from build123d import *

# Parameters (mm, degrees)
SKETCH1_R           = 14.2875
BOSS_EXTRUDE1_DEPTH = 3.9751
SKETCH2_R           = 12.7
SKETCH2_R_2         = 8.73125
CUT_EXTRUDE1_DEPTH  = 0.508


with BuildPart() as part:
    # Sketch1 → Boss-Extrude1 (new body, symmetric)
    with BuildSketch(Plane.XY):
        Circle(SKETCH1_R)
        Polygon((7.332348419, 0), (3.666174209, 6.35), (-3.666174209, 6.35), (-7.332348419, 0), (-3.666174209, -6.35), (3.666174209, -6.35), align=None, mode=Mode.SUBTRACT)
    extrude(amount=BOSS_EXTRUDE1_DEPTH, both=True)

    # Sketch2 → Cut-Extrude1 (cut)
    with BuildSketch(Plane.XY.offset(3.9751)):
        Circle(SKETCH2_R)
        Circle(SKETCH2_R_2, mode=Mode.SUBTRACT)
    cut_extrude1 = extrude(amount=-CUT_EXTRUDE1_DEPTH, mode=Mode.SUBTRACT)

    # Mirror1: Cut-Extrude1 across plane
    add(cut_extrude1.mirror(Plane.XY), mode=Mode.SUBTRACT)


solid = part.part
For this review, take the finished solid that the model builds, in its own axes (mm). A direction names the side the tool comes from. Round coordinates to 2 decimals unless told otherwise and drop trailing zeros. Order: outer loops, then holes, each group sorted by start corner. A loop starts at its lowest first (then second) coordinate and runs counter-clockwise, first axis right, second up. Notation, with made-up numbers: M 71.25,40 L 102.25,40 A17 cw 102.25,51 Z; hole C 25.5,65 d8. An arc over 180 degrees is marked long. Write each question's results on one line, items separated by ' | '. Start each with the question number.
1. To check wall thickness, follow L1, parallel to Y at x = 0, z = 3.85; L2, parallel to Y at x = 0, z = -0.25; L3, parallel to X at y = 2.25, z = -3.5. State the ranges of each line that lie inside material, in increasing order. Write a range as [from, to].
2. Clearance check with flat-ended pins moving along their axes: pin 1 Ø4 at (y, z) = (-3.5, -2.5) entering from -X; pin 2 Ø3 at (x, z) = (-9, -1) entering from -Y. State where each tip first meets the part, or that it passes through.
3. Draft analysis for pull direction Y (two halves, no side actions). For faces 4 (the face through (0, -6.35, 0)), 5 (the face through (5.1, -4.5, -3.975)), 6 (the face through (-14.274, 0.628, 0.056)), state which applies: pulls with the +Y half, pulls with the -Y half, needs draft (parallel to the pull), parting line crosses it, or undercut.
4. Add section A-A (x = 0). State the section outline as (y, z) points.
5. Add section C-C (y = 0.75). State the section outline as (x, z) points, then the cut area to 3 significant figures.
6. Tool access review of faces 1 (the face through (3, 9, 3.467)), 2 (the face through (3, 9, -3.467)), 3 (the face through (-5.474, 3.219, 0.056)): name each direction out of +Z, -Z, +X, -X, +Y, -Y from which nothing blocks a thin tool from reaching the whole face with its end or side.
7. Add section D-D (x = 9.5). State the section outline as (y, z) points, then the cut area to 3 significant figures.
Output values:
1) L1: [-14.29, -12.7], [-8.73, -6.35], [6.35, 8.73], [12.7, 14.29] | L2: [-14.29, -6.35], [6.35, 14.29] | L3: [-14.11, -12.5], [-8.44, -6.03], [6.03, 8.44], [12.5, 14.11]
2) pin 1: x = -14.21 | pin 2: y = -12.16
3) face 4: undercut | face 5: needs draft | face 6: parting line crosses it
4) outline: M -14.29,-3.98 L -12.7,-3.98 L -12.7,-3.47 L -8.73,-3.47 L -8.73,-3.98 L -6.35,-3.98 L -6.35,3.98 L -8.73,3.98 L -8.73,3.47 L -12.7,3.47 L -12.7,3.98 L -14.29,3.98 Z; M 6.35,-3.98 L 8.73,-3.98 L 8.73,-3.47 L 12.7,-3.47 L 12.7,-3.98 L 14.29,-3.98 L 14.29,3.98 L 12.7,3.98 L 12.7,3.47 L 8.73,3.47 L 8.73,3.98 L 6.35,3.98 Z
5) outline: M -14.27,-3.98 L -12.68,-3.98 L -12.68,-3.47 L -8.7,-3.47 L -8.7,-3.98 L -6.9,-3.98 L -6.9,3.98 L -8.7,3.98 L -8.7,3.47 L -12.68,3.47 L -12.68,3.98 L -14.27,3.98 Z; M 6.9,-3.98 L 8.7,-3.98 L 8.7,-3.47 L 12.68,-3.47 L 12.68,-3.98 L 14.27,-3.98 L 14.27,3.98 L 12.68,3.98 L 12.68,3.47 L 8.7,3.47 L 8.7,3.98 L 6.9,3.98 Z | area: 109 mm^2
6) face 1: +Z | face 2: -Z | face 3: +Z, -Z
7) outline: M -10.67,-3.98 L -8.43,-3.98 L -8.43,-3.47 L 8.43,-3.47 L 8.43,-3.98 L 10.67,-3.98 L 10.67,3.98 L 8.43,3.98 L 8.43,3.47 L -8.43,3.47 L -8.43,3.98 L -10.67,3.98 Z | area: 153 mm^2
